For this review, take the finished solid that the model builds, in its own axes (mm). A direction names the side the tool comes from. Round coordinates to 2 decimals unless told otherwise and drop trailing zeros. Loops run counter-clockwise (first coordinate to the right, second up) from the corner with the lowest first, then second, coordinate; pieces in that order, holes last. Notation, with made-up numbers: (71, 45.5) -> (80, 45.5) arc R26 ccw to (80, 75.5) -> close; hole circle Ø7 at (-15.5, 43). An arc over 180 degrees is marked (long way). One line per question, with ' | ' between items. Start each with the question number.
1. Draft analysis for pull direction X (two halves, no side actions). For faces 4 (the face through (12, 28, 0)), 5 (the face through (10.63, 16, 5)), 6 (the face through (0, 2, -3.085)), state which applies: pulls with the +X half, pulls with the -X half, needs draft (parallel to the pull), parting line crosses it, or undercut.
2. Consider section D-D (z = 0). Write out the cut boundary in (x, y) (3 decimals).
3. For pin 1 Ø2.5 at (y, z) = (25.5, 8) entering from -X; pin 2 Ø7 at (x, z) = (-3.5, 0.5) entering from +Y; pin 3 Ø2.5 at (x, z) = (-11, 9) entering from +Y, all flat-tipped, find the tip position at first contact; note any pin that passes through.
4. Consider section C-C (z = -8). Write out the cut boundary in (x, y), and give its area (3 significant figures).
5. Consider section A-A (x = -0.5). Write out the cut boundary in (y, z) (3 decimals).
6. Consider section B-B (y = 12.25). Write out the cut boundary in (x, z) (3 decimals).
7. Wall thickness on line 1 along Z through (x, y) = (3.5, 4); line 2 along Z through (x, y) = (-2.25, 3.25) (3 decimals); line 3 along X through (y, z) = (23.75, -3): over which ranges is each line inside the solid? List them lowest first.
8. For faces 1 (the face through (7.084, 1.652, -0.068)), 2 (the face through (-12, 6, 8)), 3 (the face through (-2, 3.35, -5)), list the 3-axis set-ups (+Z, -Z, +X, -X, +Y, -Y) from which the entire face can be reached by the end or side of a thin tool; tool diameter is ignored.
```python
from build123d import *

# Parameters (mm, degrees)
SKETCH_1_W      = 28
SKETCH_1_H      = 19.9
EXTRUDE_1_DEPTH = 3.35
SKETCH_3_W      = 22
SKETCH_3_H      = 3.35
SKETCH_3_W_2    = 6
SKETCH_3_H_2    = 2.65
EXTRUDE_2_DEPTH = 3.1
EXTRUDE_START   = -16.8
SKETCH_3_3_W    = 6
SKETCH_3_3_H    = 2.65
SKETCH_3_3_H_2  = 3.35
SKETCH_3_3_W_2  = 22
EXTRUDE_3_DEPTH = 3.1
SKETCH_4_W      = 19.9
SKETCH_4_H      = 28
EXTRUDE_4_DEPTH = 3.37


with BuildPart() as part:
    # Sketch 1 → Extrude 1 (new body)
    with BuildSketch(Plane(origin=(0, 0, 0), x_dir=(1, 0, 0), z_dir=(0, 1, 0))):
        Rectangle(SKETCH_1_W, SKETCH_1_H)
        with BuildLine():
            Line((-4, 3.085), (4, 3.085))
            ThreePointArc((4, 3.085), (7.085, 0), (4, -3.085))
            Line((4, -3.085), (-4, -3.085))
            ThreePointArc((-4, -3.085), (-7.085, 0), (-4, 3.085))
        make_face(mode=Mode.SUBTRACT)
    extrude(amount=EXTRUDE_1_DEPTH)

    # Sketch 3 → Extrude 2 (add)
    with BuildSketch(Plane.XY.offset(9.95)):
        Polygon((8, 6), (14, 6), (14, 28), (8, 28), (8, 23.2), align=None)
        Polygon((-9.2, 6), (8, 6), (8, 23.2), align=None)
        Polygon((-14, 3.35), (8, 3.35), (8, 6), (-9.2, 6), (-14, 6), align=None)
        with Locations((-3, 1.675)):
            Rectangle(SKETCH_3_W, SKETCH_3_H)
        with Locations((11, 4.675)):
            Rectangle(SKETCH_3_W_2, SKETCH_3_H_2)
        with Locations((11, 1.675)):
            Rectangle(SKETCH_3_W_2, SKETCH_3_H)
    extrude(amount=-EXTRUDE_2_DEPTH)

    # Sketch 3_3 → Extrude 3 (add)
    with BuildSketch(Plane.XY.offset(9.95).offset(EXTRUDE_START)):
        Polygon((8, 6), (14, 6), (14, 28), (8, 28), (8, 23.2), align=None)
        Polygon((-14, 3.35), (8, 3.35), (8, 6), (-9.2, 6), (-14, 6), align=None)
        with Locations((11, 4.675)):
            Rectangle(SKETCH_3_3_W, SKETCH_3_3_H)
        with Locations((11, 1.675)):
            Rectangle(SKETCH_3_3_W, SKETCH_3_3_H_2)
        with Locations((-3, 1.675)):
            Rectangle(SKETCH_3_3_W_2, SKETCH_3_3_H_2)
        Polygon((-9.2, 6), (8, 6), (8, 23.2), align=None)
    extrude(amount=-EXTRUDE_3_DEPTH)

    # Sketch 4 → Extrude 4 (add)
    with BuildSketch(Plane(origin=(14, 0, 0), x_dir=(0, 0, -1), z_dir=(1, 0, 0))):
        with Locations((0, 14)):
            Rectangle(SKETCH_4_W, SKETCH_4_H)
        with BuildLine():
            Line((3.085, 18), (3.085, 10))
            ThreePointArc((3.085, 10), (0, 6.915), (-3.085, 10))
            Line((-3.085, 10), (-3.085, 18))
            ThreePointArc((-3.085, 18), (0, 21.085), (3.085, 18))
        make_face(mode=Mode.SUBTRACT)
    extrude(amount=-EXTRUDE_4_DEPTH)


solid = part.part
```
Answer block:
1) face 4: needs draft | face 5: pulls with the -X half | face 6: undercut
2) outline: (-14, 0) -> (-7.085, 0) -> (-7.085, 3.35) -> (-14, 3.35) -> close; (7.085, 0) -> (14, 0) -> (14, 6.915) -> (10.63, 6.915) -> (10.63, 3.35) -> (7.085, 3.35) -> close; (10.63, 21.085) -> (14, 21.085) -> (14, 28) -> (10.63, 28) -> close
3) pin 1: stops at x = 8 | pin 2: stops at y = 3.35 | pin 3: stops at y = 6
4) outline: (-14, 0) -> (14, 0) -> (14, 28) -> (8, 28) -> (8, 23.2) -> (-9.2, 6) -> (-14, 6) -> close | area: 448 mm2
5) outline: (0, -9.95) -> (14.7, -9.95) -> (14.7, -6.85) -> (3.35, -6.85) -> (3.35, -3.085) -> (0, -3.085) -> close; (0, 3.085) -> (3.35, 3.085) -> (3.35, 6.85) -> (14.7, 6.85) -> (14.7, 9.95) -> (0, 9.95) -> close
6) outline: (-2.95, -9.95) -> (14, -9.95) -> (14, -3.085) -> (10.63, -3.085) -> (10.63, -6.85) -> (-2.95, -6.85) -> close; (-2.95, 6.85) -> (10.63, 6.85) -> (10.63, 3.085) -> (14, 3.085) -> (14, 9.95) -> (-2.95, 9.95) -> close
7) line 1: z = -9.95 to -6.85, 6.85 to 9.95 | line 2: z = -9.95 to -3.085, 3.085 to 9.95 | line 3: x = 10.63 to 14
8) face 1: +Y, -Y | face 2: +Z, -Z, -X, +Y | face 3: -X, +Y
